```python
from build123d import *

# Parameters (mm, degrees)
SKETCH1_W           = 27
SKETCH1_H           = 20
BOSS_EXTRUDE1_DEPTH = 50
SKETCH2_W           = 19
SKETCH2_H           = 14
BOSS_EXTRUDE2_DEPTH = 2
SKETCH3_W           = 23
SKETCH3_H           = 2
CUT_EXTRUDE1_DEPTH  = 48
SKETCH4_W           = 0.5
SKETCH4_H           = 9
SKETCH4_W_2         = 19
SKETCH4_H_2         = 0.5
BOSS_EXTRUDE3_DEPTH = 48
FILLET1_R           = 3
CUT_EXTRUDE6_REACH  = 62.241
SKETCH7_W           = 47
SKETCH7_H           = 20
BOSS_EXTRUDE5_DEPTH = 6
CUT_EXTRUDE7_REACH  = 36.132
SKETCH9_R           = 1
BOSS_EXTRUDE6_DEPTH = 6
CUT_EXTRUDE8_DEPTH  = 3


with BuildPart() as part:
    # Sketch1 → Boss-Extrude1 (new body)
    with BuildSketch(Plane.XY):
        with Locations((13.5, 10)):
            Rectangle(SKETCH1_W, SKETCH1_H)
        Polygon((4, 17), (23, 17), (23, 16), (23, 4), (23, 3), (4, 3), (4, 4), (4, 16), align=None, mode=Mode.SUBTRACT)
    extrude(amount=-BOSS_EXTRUDE1_DEPTH)

    # Sketch2 → Boss-Extrude2 (add)
    with BuildSketch(Plane(origin=(0, 0, -50), x_dir=(-1, 0, 0), z_dir=(0, 0, -1))):
        with Locations((-13.5, 10)):
            Rectangle(SKETCH2_W, SKETCH2_H)
    extrude(amount=-BOSS_EXTRUDE2_DEPTH)

    # Sketch3 → Cut-Extrude1 (cut)
    with BuildSketch(Plane.XY):
        with Locations((13.5, 13)):
            Rectangle(SKETCH3_W, SKETCH3_H)
    extrude(amount=-CUT_EXTRUDE1_DEPTH, mode=Mode.SUBTRACT)

    # Sketch4 → Boss-Extrude3 (add)
    with BuildSketch(Plane.XY):
        with Locations((4.25, 7.5)):
            Rectangle(SKETCH4_W, SKETCH4_H)
        with Locations((22.75, 7.5)):
            Rectangle(SKETCH4_W, SKETCH4_H)
        with Locations((13.5, 16.75)):
            Rectangle(SKETCH4_W_2, SKETCH4_H_2)
    extrude(amount=-BOSS_EXTRUDE3_DEPTH)

    # Fillet1
    fillet1_edges = [part.edges().sort_by_distance(p)[0] for p in [
        (0, 0, -25),
        (0, 20, -25),
        (27, 20, -25),
        (27, 0, -25),
    ]]
    fillet(fillet1_edges, radius=FILLET1_R)

    # Sketch7 → Cut-Extrude6 (cut, up to next)
    with BuildSketch(Plane(origin=(27, 0, 0), x_dir=(0, 0, -1), z_dir=(1, 0, 0)), mode=Mode.PRIVATE) as cut_extrude6_sk1:
        with Locations((26.5, 10)):
            Rectangle(SKETCH7_W, SKETCH7_H)
    cut_extrude6_tool1 = extrude(cut_extrude6_sk1.sketch, amount=-CUT_EXTRUDE6_REACH, mode=Mode.PRIVATE) & part.part
    add(cut_extrude6_tool1.solids().sort_by_distance((27, 10, -26.5))[0], mode=Mode.SUBTRACT)

    # Sketch5 → Boss-Extrude5 (add)
    with BuildSketch(Plane.XY):
        Polygon((22.5, 3), (4.5, 3), (4.5, 12), (2, 12), (2, 14), (4, 14), (4, 16.5), (23, 16.5), (23, 14), (25, 14), (25, 12), (22.5, 12), align=None)
    extrude(amount=-BOSS_EXTRUDE5_DEPTH)

    # Sketch8 → Cut-Extrude7 (cut, up to next)
    with BuildSketch(Plane(origin=(0, 0, -6), x_dir=(-1, 0, 0), z_dir=(0, 0, -1)), mode=Mode.PRIVATE) as cut_extrude7_sk1:
        with BuildLine():
            Line((-17.5, 17.5), (-9.5, 17.5))
            ThreePointArc((-9.5, 17.5), (-7, 15), (-9.5, 12.5))
            Line((-9.5, 12.5), (-17.5, 12.5))
            ThreePointArc((-17.5, 12.5), (-20, 15), (-17.5, 17.5))
        make_face()
    cut_extrude7_tool1 = extrude(cut_extrude7_sk1.sketch, amount=-CUT_EXTRUDE7_REACH, mode=Mode.PRIVATE) & part.part
    add(cut_extrude7_tool1.solids().sort_by_distance((13.5, 15, -6))[0], mode=Mode.SUBTRACT)

    # Sketch9 → Boss-Extrude6 (add)
    with BuildSketch(Plane(origin=(0, 0, -3), x_dir=(-1, 0, 0), z_dir=(0, 0, -1))):
        with Locations(Location((-24, 17, 0), (0, 0, 270))):
            Circle(SKETCH9_R)
        with Locations(Location((-3, 17, 0), (0, 0, 270))):
            Circle(SKETCH9_R)
        with Locations(Location((-3, 3, 0), (0, 0, 270))):
            Circle(SKETCH9_R)
        with Locations(Location((-24, 3, 0), (0, 0, 270))):
            Circle(SKETCH9_R)
    extrude(amount=BOSS_EXTRUDE6_DEPTH)

    # Sketch11 → Cut-Extrude8 (cut)
    with BuildSketch(Plane(origin=(0, 0, -6), x_dir=(-1, 0, 0), z_dir=(0, 0, -1))):
        with BuildLine():
            ThreePointArc((-7.5, 16.5), (-7.263932023, 13.881966011), (-9.5, 12.5))
            Line((-9.5, 12.5), (-17.5, 12.5))
            ThreePointArc((-17.5, 12.5), (-19.736067977, 13.881966011), (-19.5, 16.5))
            Line((-19.5, 16.5), (-23, 16.5))
            Line((-23, 16.5), (-23, 14))
            Line((-23, 14), (-25, 14))
            Line((-25, 14), (-25, 12))
            Line((-25, 12), (-22.5, 12))
            Line((-22.5, 12), (-22.5, 3))
            Line((-22.5, 3), (-4.5, 3))
            Line((-4.5, 3), (-4.5, 12))
            Line((-4.5, 12), (-2, 12))
            Line((-2, 12), (-2, 14))
            Line((-2, 14), (-4, 14))
            Line((-4, 14), (-4, 16.5))
            Line((-4, 16.5), (-7.5, 16.5))
        make_face()
        with BuildLine():
            Line((-20.029822128, 16.2), (-22.7, 16.2))
            Line((-22.7, 16.2), (-22.7, 13.7))
            Line((-22.7, 13.7), (-24.7, 13.7))
            Line((-24.7, 13.7), (-24.7, 12.3))
            Line((-24.7, 12.3), (-22.2, 12.3))
            Line((-22.2, 12.3), (-22.2, 3.3))
            Line((-22.2, 3.3), (-4.8, 3.3))
            Line((-4.8, 3.3), (-4.8, 12.3))
            Line((-4.8, 12.3), (-2.3, 12.3))
            Line((-2.3, 12.3), (-2.3, 13.7))
            Line((-2.3, 13.7), (-4.3, 13.7))
            Line((-4.3, 13.7), (-4.3, 16.2))
            Line((-4.3, 16.2), (-6.970177872, 16.2))
            ThreePointArc((-6.970177872, 16.2), (-7.133568087, 13.503337045), (-9.5, 12.2))
            Line((-9.5, 12.2), (-17.5, 12.2))
            ThreePointArc((-17.5, 12.2), (-19.866431913, 13.503337045), (-20.029822128, 16.2))
        make_face(mode=Mode.SUBTRACT)
    extrude(amount=-CUT_EXTRUDE8_DEPTH, mode=Mode.SUBTRACT)


solid = part.part
```
Geometry check sheet. Reference: the model listing, model coordinates, mm. A direction names the side the tool comes from. Give positions to 0.01 mm unless a question says otherwise; leave off trailing zeros. Loops run counter-clockwise (first coordinate to the right, second up) from the corner with the lowest first, then second, coordinate; pieces in that order, holes last. Notation, with made-up numbers: M 28,65 L 45,65 A28 cw 45,97 Z; hole C -6.5,-11.75 d1. An arc over 180 degrees is marked long. Answer as CSV lines item,"result".
Item 1: Access from +Z, -Z, +X, -X, +Y, -Y to the whole of each face (thin tool, end or side, straight path). Record for faces 4 (the cylindrical face through (20, 15, -2)), 5 (the flat face through (23, 12.3, -5)), 6 (the flat face through (6, 16.2, -5)), 7 (the flat face through (14, 3.3, -5)).
Values:
face 4,"+Z, -Z"
face 5,"-Z, +X"
face 6,"-Z, +Y"
face 7,"-Z, -Y"
Item 2: Release check for a two-part mould opening along X. For faces 1 (the flat face through (24, 3, -9)), 2 (the flat face through (13, 12.2, -5)), 3 (the flat face through (2.3, 13, -5)) record: pulls with the +X half, pulls with the -X half, needs draft (parallel to the pull), parting line crosses it, or undercut.
Values:
face 1,"needs draft"
face 2,"undercut"
face 3,"pulls with the -X half"
Item 3: Depth check by flat-ended pin: P1, Ø0.8, axis at x = 23.5, z = -4, coming from the -Y side (3 decimals); P2, Ø4, axis at x = 14.5, y = 6.5, coming from the -Z side; P3, Ø2.5, axis at x = 11.5, z = -4.5, coming from the -Y side; P4, Ø2, axis at x = 4.5, y = 3.5, coming from the -Z side. Enter the tip coordinate at first touch or a pass-through.
Values:
P1,"stops at y = 2.005"
P2,"stops at z = -6"
P3,"stops at y = 3.3"
P4,"stops at z = -9"
Item 4: Cross-section at C-C on z = -1.75. Record the cut outline in (x, y), and give its area (3 significant figures).
Values:
outline,"M 0,3 A3 ccw 3,0 L 24,0 A3 ccw 27,3 L 27,17 A3 ccw 24,20 L 3,20 A3 ccw 0,17 Z; hole M 9.5,12.5 L 17.5,12.5 A2.5 ccw 17.5,17.5 L 9.5,17.5 A2.5 ccw Z"
area,"473 mm²"
Item 5: Cross-section at B-B on z = -4. Record the cut outline in (x, y), and give its area (3 significant figures).
Values:
outline,"C 3,3 d2; C 3,17 d2; M 2.3,12.3 L 4.8,12.3 L 4.8,3.3 L 22.2,3.3 L 22.2,12.3 L 24.7,12.3 L 24.7,13.7 L 22.7,13.7 L 22.7,16.2 L 20.03,16.2 A2.8 cw 17.5,12.2 L 9.5,12.2 A2.8 cw 6.97,16.2 L 4.3,16.2 L 4.3,13.7 L 2.3,13.7 Z; C 24,3 d2; C 24,17 d2"
area,"196 mm²"
Item 6: Cross-section at D-D on y = 7. Record the cut outline in (x, z).
Values:
outline,"M 0,-3 L 4.8,-3 L 4.8,-6 L 22.2,-6 L 22.2,-3 L 27,-3 L 27,0 L 0,0 Z"
Item 7: Cross-section at A-A on x = 10.25. Record the cut outline in (y, z), and give its area (3 significant figures).
Values:
outline,"M 0,-3 L 3.3,-3 L 3.3,-6 L 12.2,-6 L 12.2,-3 L 12.5,-3 L 12.5,0 L 0,0 Z; M 17.5,-3 L 20,-3 L 20,0 L 17.5,0 Z"
area,"71.7 mm²"
Item 8: Material ranges on line 1 (Y direction, x = 16.75, z = -2.75); line 2 (X direction, y = 13.75, z = -4.25); line 3 (Y direction, x = 3.5, z = -4), recorded low to high.
Values:
line 1,"y = 0 to 12.5, 17.5 to 20"
line 2,"x = 4.3 to 6.99, 20.01 to 22.7"
line 3,"y = 2.13 to 3.87, 12.3 to 13.7, 16.13 to 17.87"
